Check sheet for the drawn part. Datum: minimum x, y, z corner. Units: mm. A direction names the side the tool comes from. Coordinates: 2 decimals unless noted, no trailing zeros. Write each loop counter-clockwise with the first axis right and the second up, starting at its lowest first coordinate (ties: lowest second). Pieces come first, ordered by that corner, then holes. Notation, with made-up numbers: (52, -3.75) -> (109, -3.75) arc R17 cw to (109, 19.25) -> close; hole circle Ø11 at (-8, -11). An arc over 180 degrees is marked (long way). Write each question's results on one line, items separated by ' | '. Start each with the question number.
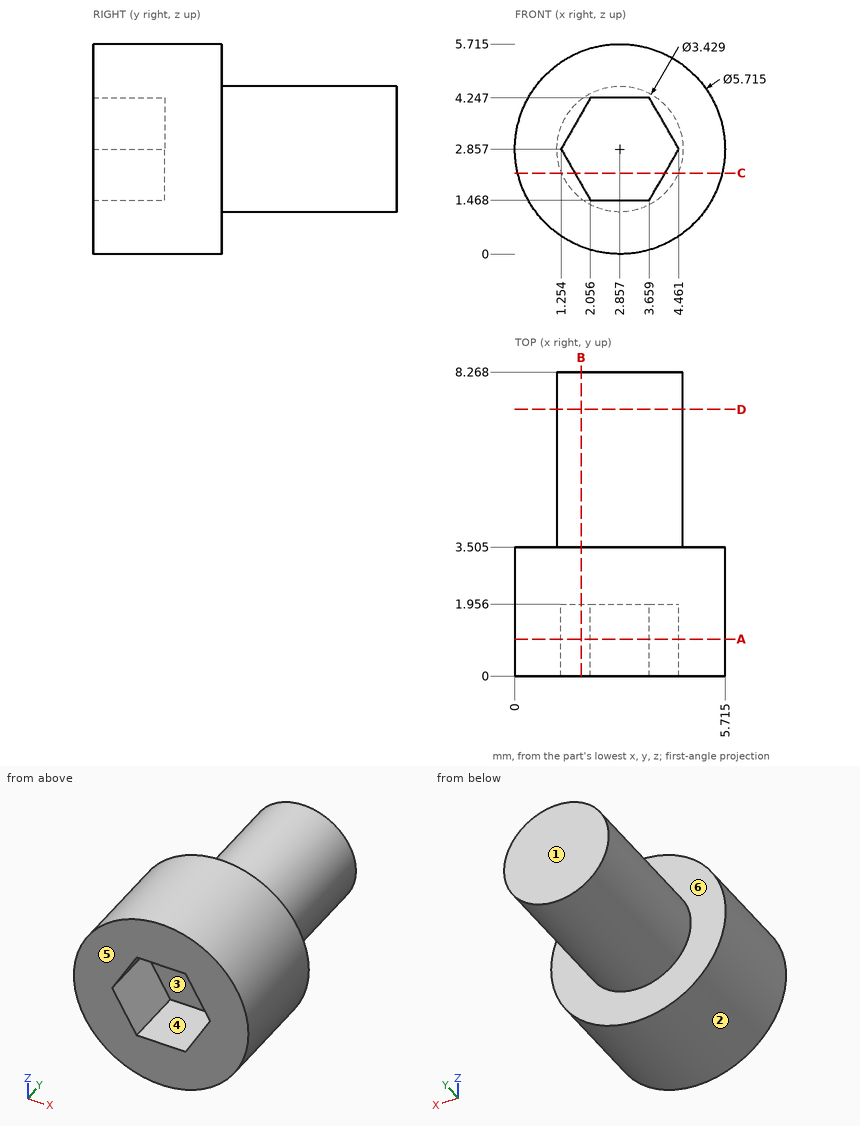
1. Mould release check, pull along X, two halves, no side actions. Record for the marked faces 1, 2 and 3: +X half, -X half, draft (parallel to the pull), parting line (faces both ways), or undercut.
2. Material ranges on probe 1 along Y at (x, z) = (2.55, 4.95) (1 decimal); probe 2 along X at (y, z) = (4.5, 2.85); probe 3 along X at (y, z) = (8, 4) (1 decimal), recorded low to high. Write a range as from..to.
3. Sectioned sample at A-A on y = 1. Record the cut outline in (x, z) (1 decimal).
4. Sectioned sample at B-B on x = 1.8. Record the cut outline in (y, z) (1 decimal).
5. Depth check by flat-ended pin: pin 1 Ø1.4 at (x, z) = (3, 2.5) entering from -Y; pin 2 Ø1.5 at (y, z) = (3.5, 2) entering from +X; pin 3 Ø1.3 at (x, y) = (3, 1) entering from -Z; pin 4 Ø3 at (x, y) = (0.5, 2) entering from -Z. Enter the tip coordinate at first touch or a pass-through.
6. Sectioned sample at C-C on z = 2.2. Record the cut outline in (x, y) (1 decimal).
7. Tool access check on the marked faces 4, 5 and 6. Record the directions out of +Z, -Z, +X, -X, +Y, -Y that give a thin tool (end or side, any length) a straight path to the whole face; none if there is none.
8. Sectioned sample at D-D on y = 7.25. Record the cut outline in (x, z) (1 decimal).
Computed values:
1) face 1: draft | face 2: parting line | face 3: undercut
2) probe 1: y = 0..3.5 | probe 2: x = 1.14..4.57 | probe 3: x = 1.6..4.1
3) outline: circle Ø5.7 at (2.9, 2.9); hole (1.3, 2.9) -> (2.1, 1.5) -> (3.7, 1.5) -> (4.5, 2.9) -> (3.7, 4.2) -> (2.1, 4.2) -> close
4) outline: (0, 0.2) -> (3.5, 0.2) -> (3.5, 1.5) -> (8.3, 1.5) -> (8.3, 4.2) -> (3.5, 4.2) -> (3.5, 5.5) -> (0, 5.5) -> (0, 3.8) -> (2, 3.8) -> (2, 1.9) -> (0, 1.9) -> close
5) pin 1: stops at y = 1.96 | pin 2: stops at x = 5.71 | pin 3: stops at z = 0 | pin 4: stops at z = 0.13
6) outline: (0.1, 0) -> (1.6, 0) -> (1.6, 2) -> (4.1, 2) -> (4.1, 0) -> (5.6, 0) -> (5.6, 3.5) -> (4.4, 3.5) -> (4.4, 8.3) -> (1.3, 8.3) -> (1.3, 3.5) -> (0.1, 3.5) -> close
7) face 4: -Y | face 5: +Z, -Z, +X, -X, -Y | face 6: +Y
8) outline: circle Ø3.4 at (2.9, 2.9)
